Here's the drawing with two shaded views (mm, measured from the low corner). I have some questions. Coordinates: 2 decimals unless noted, no trailing zeros. Write each loop counter-clockwise with the first axis right and the second up, starting at its lowest first coordinate (ties: lowest second). Pieces come first, ordered by that corner, then holes.
Item 1: If we section it at A-A (x = 13.97): Please give me the cut outline in (y, z).
Item 2: I'm going to push flat-ended pins straight in: pin 1 Ø1.5 at (x, z) = (5, 7.5) entering from +Y; pin 2 Ø0.6 at (y, z) = (3, 11) entering from +X (1 decimal); pin 3 Ø0.8 at (y, z) = (2.5, 10) entering from -X. Where does each tip first touch, or does it pass through?
Item 3: If I drill on line 1 (Z direction, x = 11.43, y = 0.8); line 2 (Z direction, x = 19.05, y = 0.45); line 3 (X direction, y = 1, z = 3.81), over which ranges is the centre line in solid material (lowest first)?
Item 4: If we section it at C-C (z = 6.35): Please give me the cut outline in (x, y).
Item 5: If we section it at B-B (y = 1.3): Count the separate pieces of the cut face and the enclosed holes in it, then the cut area to 3 significant figures.
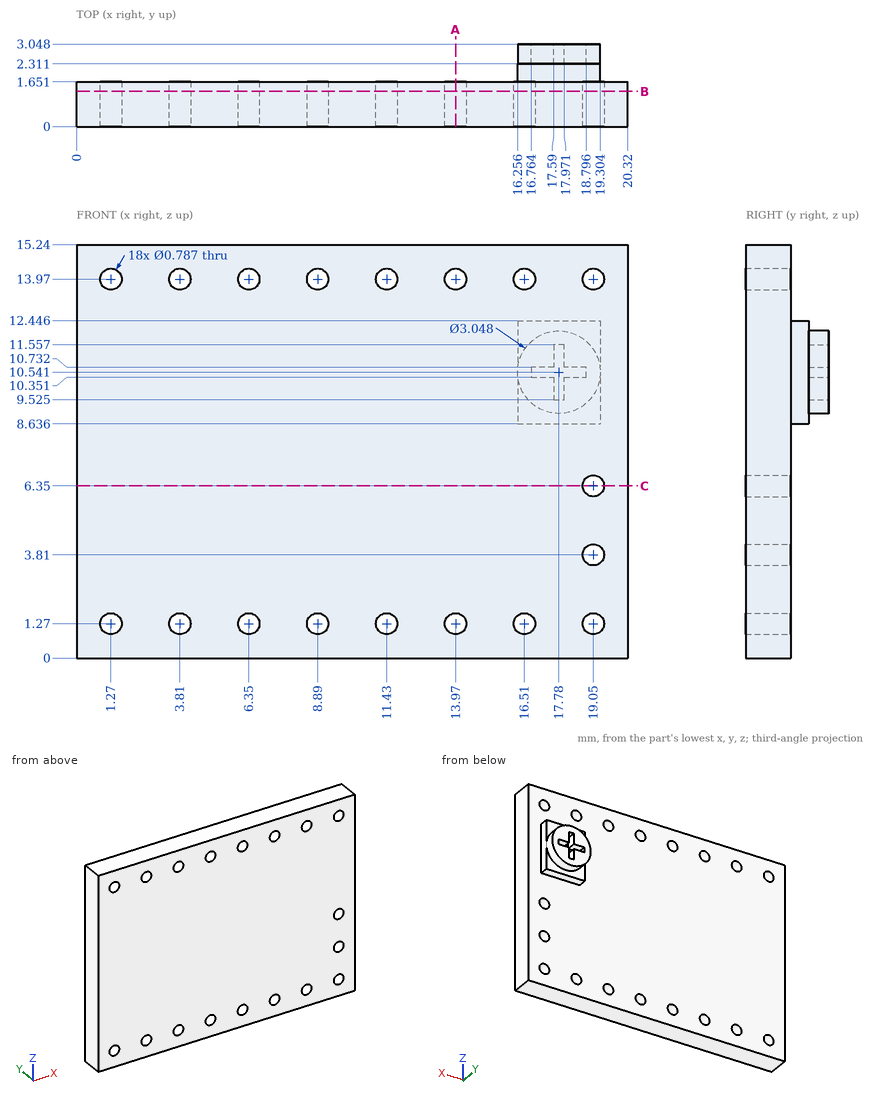
Answer list:
1. outline: (0, 0) - (1.65, 0) - (1.65, 0.88) - (0, 0.88) - close; (0, 1.66) - (1.65, 1.66) - (1.65, 13.58) - (0, 13.58) - close; (0, 14.36) - (1.65, 14.36) - (1.65, 15.24) - (0, 15.24) - close
2. pin 1: stops at y = 1.65
2. pin 2: stops at x = 19.3
2. pin 3: stops at x = 16.26
3. line 1: z = 0 to 0.88, 1.66 to 13.58, 14.36 to 15.24
3. line 2: z = 0 to 0.88, 1.66 to 3.42, 4.2 to 5.96, 6.74 to 13.58, 14.36 to 15.24
3. line 3: x = 0 to 18.66, 19.44 to 20.32
4. outline: (0, 0) - (18.66, 0) - (18.66, 1.65) - (0, 1.65) - close; (19.44, 0) - (20.32, 0) - (20.32, 1.65) - (19.44, 1.65) - close
5. separate pieces: 1
5. enclosed holes: 18
5. area: 301 mm2
